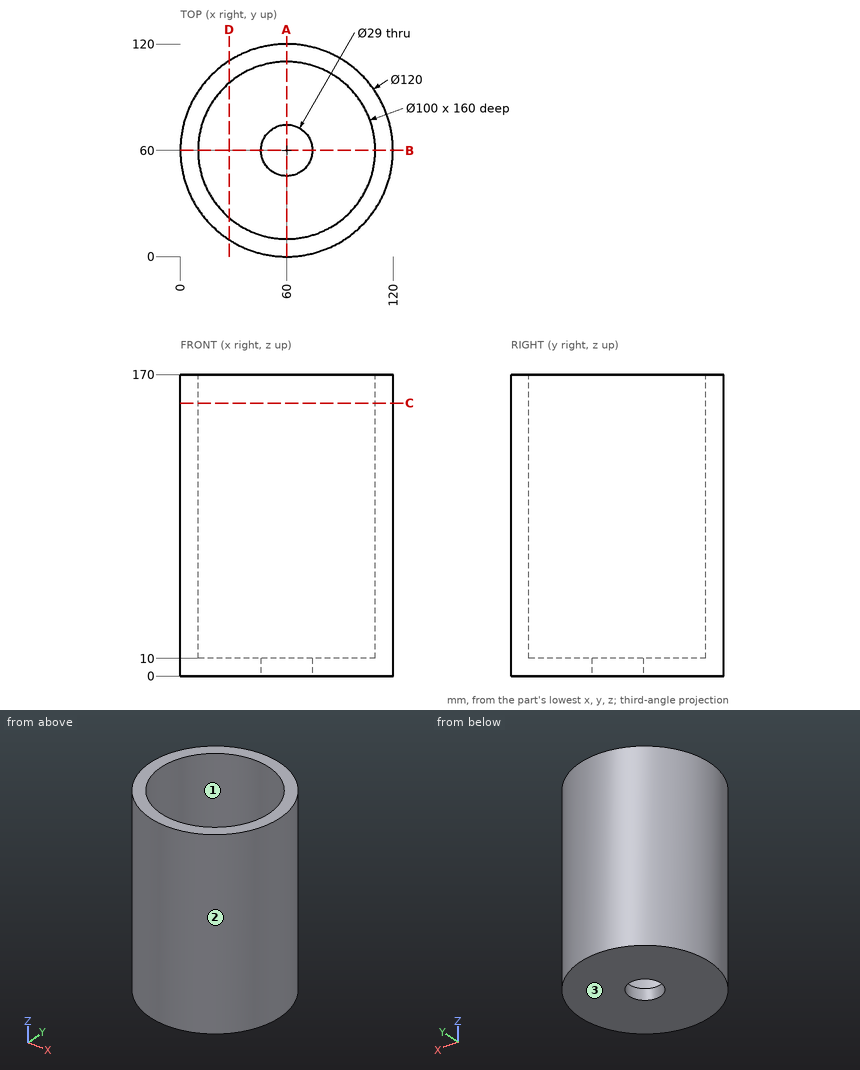
Job drawing, mm, ordinate dimensions from the low corner. One solid piece. Give positions to 0.01 mm unless a question says otherwise; leave off trailing zeros. Loops run counter-clockwise (first coordinate to the right, second up) from the corner with the lowest first, then second, coordinate; pieces in that order, holes last. Notation, with made-up numbers: M 85,47.25 L 91,47.25 A35 cw 91,84.25 Z; hole C 33.5,-18.5 d6. An arc over 180 degrees is marked long. Answer in a Markdown table with one row per item. Add a question column.
Item 1: Band-saw the part on D-D on x = 27.5. Give the cut face in (y, z).
Item 2: Band-saw the part on C-C on z = 154. Give the cut face in (x, y).
Item 3: Probe probe 1 along Y at (x, z) = (60, 2); probe 2 along Y at (x, z) = (60, 127); probe 3 along X at (y, z) = (101.5, 39.5). List the from-to ranges inside material, lowest first.
Item 4: Drop flat-ended pins along their axis: P1, Ø10, axis at y = 12, z = 141, coming from the -X side; P2, Ø10, axis at x = 67.5, z = 152.5, coming from the -Y side; P3, Ø12, axis at x = 31, z = 111.5, coming from the -Y side. Give the stop position or say it passes through.
Item 5: Mould opens along X. For the marked faces 1, 2 and 3 say: +X half, -X half, draft (parallel to the pull), parting line (faces both ways), or undercut.
Item 6: Band-saw the part on A-A on x = 60. Give the cut face in (y, z).
Reply:
| question | item | result |
|---|---|---|
| 1 | outline | M 9.56,0 L 110.44,0 L 110.44,170 L 98,170 L 98,10 L 22,10 L 22,170 L 9.56,170 Z |
| 2 | outline | C 60,60 d120; hole C 60,60 d100 |
| 3 | probe 1 | y = 0 to 45.5, 74.5 to 120 |
| 3 | probe 2 | y = 0 to 10, 110 to 120 |
| 3 | probe 3 | x = 16.67 to 32.11, 87.89 to 103.33 |
| 4 | P1 | stops at x = 18.16 |
| 4 | P2 | stops at y = 0.05 |
| 4 | P3 | stops at y = 4.58 |
| 5 | face 1 | undercut |
| 5 | face 2 | parting line |
| 5 | face 3 | draft |
| 6 | outline | M 0,0 L 45.5,0 L 45.5,10 L 10,10 L 10,170 L 0,170 Z; M 74.5,0 L 120,0 L 120,170 L 110,170 L 110,10 L 74.5,10 Z |
